```python
from build123d import *

# Parameters (mm, degrees)
SKETCH1_W           = 195
SKETCH1_H           = 85
BOSS_EXTRUDE1_DEPTH = 3
FILLET1_R           = 2.5
BOSS_EXTRUDE2_DEPTH = 6
BOSS_EXTRUDE3_DEPTH = 8
BOSS_EXTRUDE4_DEPTH = 19.5
BOSS_EXTRUDE5_DEPTH = 21.5
FILLET2_R           = 1
SKETCH7_R           = 4
BOSS_EXTRUDE6_DEPTH = 25.5
BOSS_EXTRUDE7_DEPTH = 3
BOSS_EXTRUDE8_DEPTH = 8


with BuildPart() as part:
    # Sketch1 → Boss-Extrude1 (new body)
    with BuildSketch(Plane(origin=(0, 0, 0), x_dir=(1, 0, 0), z_dir=(0, 1, 0))):
        Rectangle(SKETCH1_W, SKETCH1_H)
    extrude(amount=BOSS_EXTRUDE1_DEPTH)

    # Fillet1
    fillet1_edges = [part.edges().sort_by_distance(p)[0] for p in [
        (97.5, 1.5, 42.5),
        (-97.5, 1.5, 42.5),
        (-97.5, 1.5, -42.5),
        (97.5, 1.5, -42.5),
    ]]
    fillet(fillet1_edges, radius=FILLET1_R)

    # Sketch3 → Boss-Extrude2 (add)
    with BuildSketch(Plane(origin=(0, 3, 0), x_dir=(1, 0, 0), z_dir=(0, 1, 0))):
        with BuildLine():
            Line((82, -37.5), (4, -37.5))
            Line((4, -37.5), (3.605042507, -37.5))
            Line((3.605042507, -37.5), (-13.095926291, -33.024988898))
            Line((-13.095926291, -33.024988898), (-80.24005573, -15.033773638))
            Line((-80.24005573, -15.033773638), (-83.294095226, -14.215446222))
            ThreePointArc((-83.294095226, -14.215446222), (-85.966766701, -12.429624235), (-87, -9.38581709))
            Line((-87, -9.38581709), (-87, 27))
            ThreePointArc((-87, 27), (-85.535533906, 30.535533906), (-82, 32))
            Line((-82, 32), (-81.875932746, 32))
            Line((-81.875932746, 32), (82, 32))
            ThreePointArc((82, 32), (85.535533906, 30.535533906), (87, 27))
            Line((87, 27), (87, -32.5))
            ThreePointArc((87, -32.5), (85.535533906, -36.035533906), (82, -37.5))
        make_face()
        with BuildLine():
            Line((-84, -9.38581709), (-84, 27))
            ThreePointArc((-84, 27), (-83.414213562, 28.414213562), (-82, 29))
            Line((-82, 29), (82, 29))
            ThreePointArc((82, 29), (83.414213562, 28.414213562), (84, 27))
            Line((84, 27), (84, -32.5))
            ThreePointArc((84, -32.5), (83.414213562, -33.914213562), (82, -34.5))
            Line((82, -34.5), (4, -34.5))
            Line((4, -34.5), (-82.51763809, -11.317668743))
            ThreePointArc((-82.51763809, -11.317668743), (-83.586706681, -10.603339948), (-84, -9.38581709))
        make_face(mode=Mode.SUBTRACT)
    extrude(amount=BOSS_EXTRUDE2_DEPTH)

    # Sketch4 → Boss-Extrude3 (add)
    with BuildSketch(Plane(origin=(0, 3, 0), x_dir=(1, 0, 0), z_dir=(0, 1, 0))):
        Polygon((-35, 35.5), (-35, 32), (-36.5, 32), (-36.5, 37), (-3, 37), (-1.5, 37), (-1.5, 32), (-3, 32), (-3, 35.5), align=None)
    extrude(amount=BOSS_EXTRUDE3_DEPTH)

    # Sketch5 → Boss-Extrude4 (add)
    with BuildSketch(Plane(origin=(0, 3, 0), x_dir=(1, 0, 0), z_dir=(0, 1, 0))):
        Polygon((93.717571079, -28.970923081), (93.717571079, -19.029076919), (87.444515609, -17.040885435), (87, -16.9), (87, -18), (92.717571079, -19.66614718), (92.717571079, -28.33385282), (87, -31), (87, -32.103377919), (87.422618262, -31.906307787), align=None)
        Polygon((-71.878679656, -17.274197605), (-71.056906471, -21.934704933), (-62.363574034, -24.264076339), (-59.321643915, -20.638845191), (-58.255862687, -20.92442041), (-58.555599472, -21.281632801), (-62.007030461, -25.394888082), (-71.931088134, -22.735744843), (-72.863487409, -17.447845782), (-72.944460885, -16.988622385), align=None)
    extrude(amount=BOSS_EXTRUDE4_DEPTH)

    # Sketch6 → Boss-Extrude5 (add)
    with BuildSketch(Plane(origin=(0, 3, 0), x_dir=(1, 0, 0), z_dir=(0, 1, 0))):
        with BuildLine():
            Line((95, -35.5), (95, -14.5))
            Line((95, -14.5), (87, -14.5))
            Line((87, -14.5), (87, -13))
            Line((87, -13), (96.5, -13))
            Line((96.5, -13), (96.5, -37))
            Line((96.5, -37), (84.179449472, -37))
            ThreePointArc((84.179449472, -37), (85.179449472, -36.358898944), (86, -35.5))
            Line((86, -35.5), (95, -35.5))
        make_face()
        Polygon((-75.742382962, -16.238921424), (-78.330573413, -25.898179687), (-68.188352237, -28.615779661), (-58.046131061, -31.333379634), (-55.45794061, -21.674121371), (-54.00905187, -22.062349939), (-56.985470889, -33.170496941), (-68.576580804, -30.0646684), (-80.16769072, -26.958839859), (-77.191271701, -15.850692856), align=None)
    extrude(amount=BOSS_EXTRUDE5_DEPTH)

    # Fillet2
    fillet2_edges = [part.edges().sort_by_distance(p)[0] for p in [
        (-1.5, 7, -37),
        (-36.5, 7, -37),
        (-35, 7, -35.5),
        (-3, 7, -35.5),
        (95, 13.75, 14.5),
        (95, 13.75, 35.5),
        (96.5, 13.75, 37),
        (96.5, 13.75, 13),
        (-80.16769072, 13.75, 26.958839859),
        (-56.985470889, 13.75, 33.170496941),
        (-58.046131061, 13.75, 31.333379634),
        (-78.330573413, 13.75, 25.898179687),
    ]]
    fillet(fillet2_edges, radius=FILLET2_R)

    # Sketch7 → Boss-Extrude6 (add)
    with BuildSketch(Plane(origin=(0, 3, 0), x_dir=(1, 0, 0), z_dir=(0, 1, 0))):
        with Locations(Location((-40, 5, 0), (0, 0, 270))):
            Circle(SKETCH7_R)
    extrude(amount=BOSS_EXTRUDE6_DEPTH)

    # Sketch8 → Boss-Extrude7 (add)
    with BuildSketch(Plane(origin=(0, 3, 0), x_dir=(1, 0, 0), z_dir=(0, 1, 0))):
        with BuildLine():
            Line((24.8, 15.15), (26, 14.25))
            ThreePointArc((26, 14.25), (49, 25.75), (72, 14.25))
            Line((72, 14.25), (73.2, 15.15))
            ThreePointArc((73.2, 15.15), (49, 27.25), (24.8, 15.15))
        make_face()
        with BuildLine():
            Line((24.8, -21.15), (26, -20.25))
            ThreePointArc((26, -20.25), (49, -31.75), (72, -20.25))
            Line((72, -20.25), (73.2, -21.15))
            ThreePointArc((73.2, -21.15), (49, -33.25), (24.8, -21.15))
        make_face()
    extrude(amount=BOSS_EXTRUDE7_DEPTH)

    # Sketch9 → Boss-Extrude8 (add)
    with BuildSketch(Plane(origin=(0, 3, 0), x_dir=(1, 0, 0), z_dir=(0, 1, 0))):
        with BuildLine():
            Line((64.363989362, -27.300418327), (65.449871217, -28.386300182))
            ThreePointArc((65.449871217, -28.386300182), (65.016806514, -28.661730438), (64.579131266, -28.929773794))
            Line((64.579131266, -28.929773794), (63.484213314, -27.834855842))
            ThreePointArc((63.484213314, -27.834855842), (63.926493446, -27.571574907), (64.363989362, -27.300418327))
        make_face()
        with BuildLine():
            Line((76.19985084, -12.312927266), (77.373998096, -13.487074522))
            ThreePointArc((77.373998096, -13.487074522), (77.180097488, -13.997481782), (76.977016247, -14.504306235))
            Line((76.977016247, -14.504306235), (75.822470959, -13.349760947))
            ThreePointArc((75.822470959, -13.349760947), (76.016135348, -12.833154674), (76.19985084, -12.312927266))
        make_face()
    extrude(amount=BOSS_EXTRUDE8_DEPTH)


solid = part.part
```
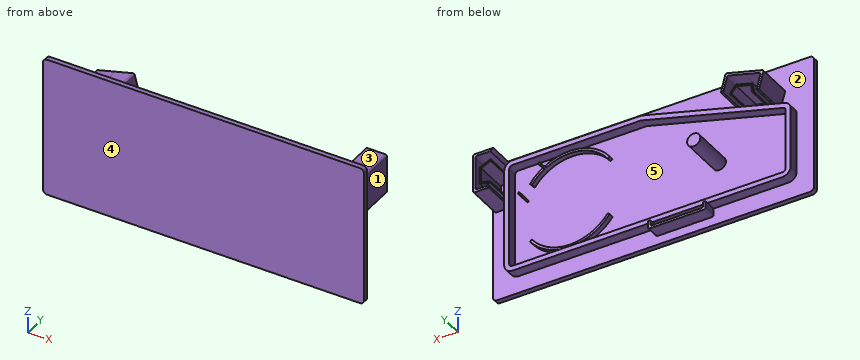
Here's how the part is built. I have some questions about the finished solid (model axes, mm). Face numbers are marked on the shaded views. A direction names the side the tool comes from. Coordinates: 2 decimals unless noted, no trailing zeros. Write each loop counter-clockwise with the first axis right and the second up, starting at its lowest first coordinate (ties: lowest second). Pieces come first, ordered by that corner, then holes. Notation, with made-up numbers: (80, 69) - (124, 69) arc R22 ccw to (124, 88) - close; hole circle Ø9 at (51, 74.5). An arc over 180 degrees is marked (long way). One line per item, written item: value.
1) Suppose I cut it at A-A on z = -5. Write out the boundary of the cut face in (x, y).
Model answer:
outline: (-97.5, 0) - (97.5, 0) - (97.5, 3) - (87, 3) - (87, 9) - (84, 9) - (84, 3) - (-36, 3) - (-36, 28.5) - (-44, 28.5) - (-44, 3) - (-84, 3) - (-84, 9) - (-87, 9) - (-87, 3) - (-97.5, 3) - close
2) Suppose I cut it at D-D on x = 7.5. Write out the boundary of the cut face in (y, z), and give its area (3 significant figures).
Model answer:
outline: (0, -42.5) - (3, -42.5) - (3, -32) - (9, -32) - (9, -29) - (3, -29) - (3, 34.5) - (9, 34.5) - (9, 37.5) - (3, 37.5) - (3, 42.5) - (0, 42.5) - close
area: 291 mm²
3) I need wall thicknesses on line 1 along Y through (x, z) = (-49, 29); line 2 along Y through (x, z) = (84.5, 10); line 3 along Z through (x, y) = (-69.5, 17.75). Which ranges of each line are inside material? Lowest first, please.
Model answer:
line 1: y = 0 to 3
line 2: y = 0 to 9
line 3: z = 22.35 to 23.39, 28.26 to 29.82
4) Suppose I cut it at C-C on y = 18.75. State how many separate pieces and enclosed holes the cut face has, and give its area (3 significant figures).
Model answer:
separate pieces: 5
enclosed holes: 0
area: 222 mm²
5) On a 3-axis mill with a long thin cutter (end or side, diameter ignored), from which of +Z, -Z, +X, -X, +Y, -Y can I reach the whole of each face in a straight line? I mean the marked faces 1 and 2. Say none if no direction works.
Model answer:
face 1: +Z, -Z, +X, +Y
face 2: +Y
6) I'm going to push flat-ended pins straight in: P1, Ø3, axis at x = -31, z = 29, coming from the +Y side; P2, Ø1.5, axis at x = -61, z = 5, coming from the +Y side; P3, Ø0.7, axis at y = 6, z = 15.5, coming from the +X side. Where does each tip first touch, or does it pass through?
Model answer:
P1: stops at y = 9
P2: stops at y = 3
P3: stops at x = 96.5
7) Suppose I cut it at B-B on x = 47.5. Write out the boundary of the cut face in (y, z), and give its area (3 significant figures).
Model answer:
outline: (0, -42.5) - (3, -42.5) - (3, -32) - (9, -32) - (9, -29) - (3, -29) - (3, -27.21) - (6, -27.21) - (6, -25.71) - (3, -25.71) - (3, 31.71) - (6, 31.71) - (6, 33.21) - (3, 33.21) - (3, 34.5) - (9, 34.5) - (9, 37.5) - (3, 37.5) - (3, 42.5) - (0, 42.5) - close
area: 300 mm²
8) We'd pull the mould along Z, two halves only. Please class the marked faces 3, 4 and 5: pulls with the +Z half, pulls with the -Z half, needs draft (parallel to the pull), parting line crosses it, or undercut.
Model answer:
face 3: pulls with the +Z half
face 4: needs draft
face 5: undercut
